For this review, use the dimensioned drawing (mm, ordinates from the lowest corner) and the shaded views. Round coordinates to 2 decimals unless told otherwise and drop trailing zeros. Loops run counter-clockwise (first coordinate to the right, second up) from the corner with the lowest first, then second, coordinate; pieces in that order, holes last. Notation, with made-up numbers: M 79,9 L 130,9 A15 cw 130,15 Z; hole C 52,-38.75 d8. An arc over 180 degrees is marked long. Answer as a JSON object with one key per item and string values. Group by question number.
Item 1: Consider section C-C (x = 39.5). Give the boundary of the cut face in (y, z), and give its area (3 significant figures).
Item 2: To check wall thickness, follow line 1 (X direction, y = 0.85, z = 23); line 2 (X direction, y = 0.2, z = 22); line 3 (Z direction, x = 2, y = 1.7). State the ranges of each line that lie inside material, in increasing order.
Item 3: Insertion check: P1, Ø6, axis at x = 17, z = 8.5, coming from the -Y side. The pin has a flat end and moves straight along its axis. Give the tip position at first contact, or say it passes through.
Item 4: Consider section A-A (y = 0.7). Give the boundary of the cut face in (x, z).
Item 5: The part is to be moulded in two halves that separate along Y. For the marked faces 1, 2 and 3, say which applies: +Y half, -Y half, draft (parallel to the pull), parting line (faces both ways), or undercut.
Item 6: Consider section B-B (z = 2.5). Give the boundary of the cut face in (x, y), and give its area (3 significant figures).
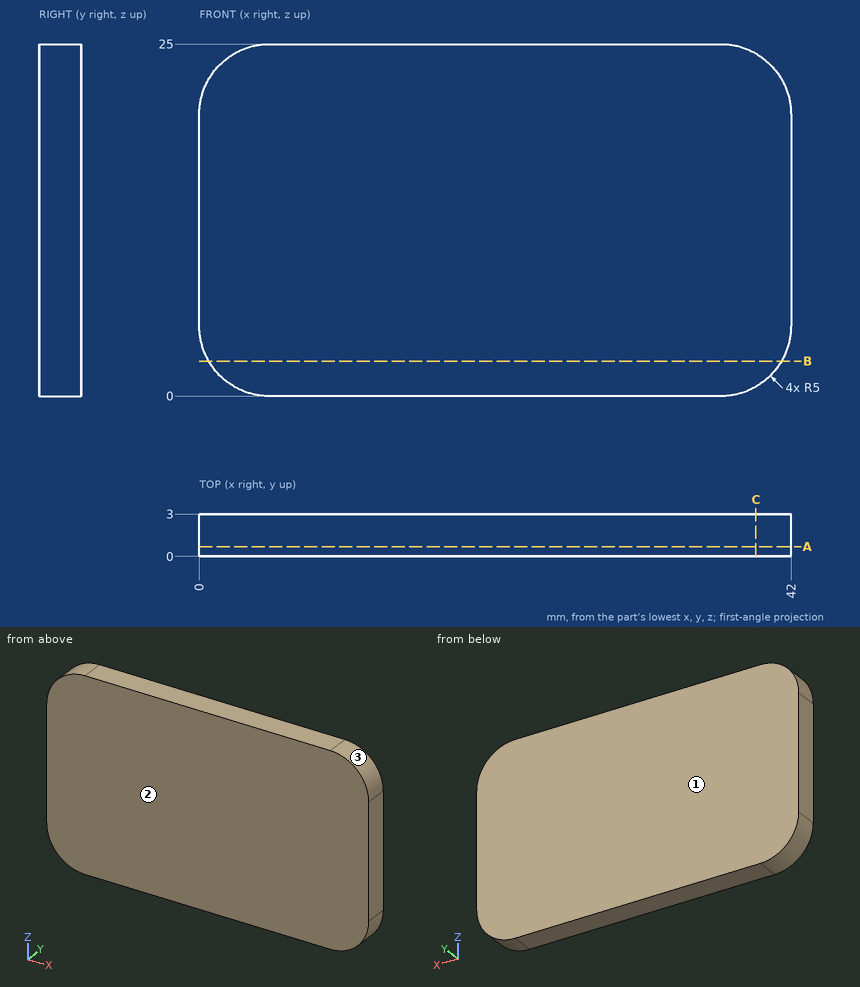
Geometry results:
{
 "1": {"outline": "M 0,0.67 L 3,0.67 L 3,24.33 L 0,24.33 Z", "area": "71.0 mm^2"},
 "2": {"line 1": "x = 1 to 41", "line 2": "x = 0.42 to 41.58", "line 3": "z = 1 to 24"},
 "3": {"P1": "stops at y = 0"},
 "4": {"outline": "M 0,5 A5 ccw 5,0 L 37,0 A5 ccw 42,5 L 42,20 A5 ccw 37,25 L 5,25 A5 ccw 0,20 Z"},
 "5": {"face 1": "+Y half", "face 2": "-Y half", "face 3": "draft"},
 "6": {"outline": "M 0.67,0 L 41.33,0 L 41.33,3 L 0.67,3 Z", "area": "122 mm^2"}
}
